Geometry: see drawing. Coordinates: mm, zero at the bounding-box minimum. A direction names the side the tool comes from. Coordinates: 2 decimals unless noted, no trailing zeros. Loops run counter-clockwise (first coordinate to the right, second up) from the corner with the lowest first, then second, coordinate; pieces in that order, holes last.
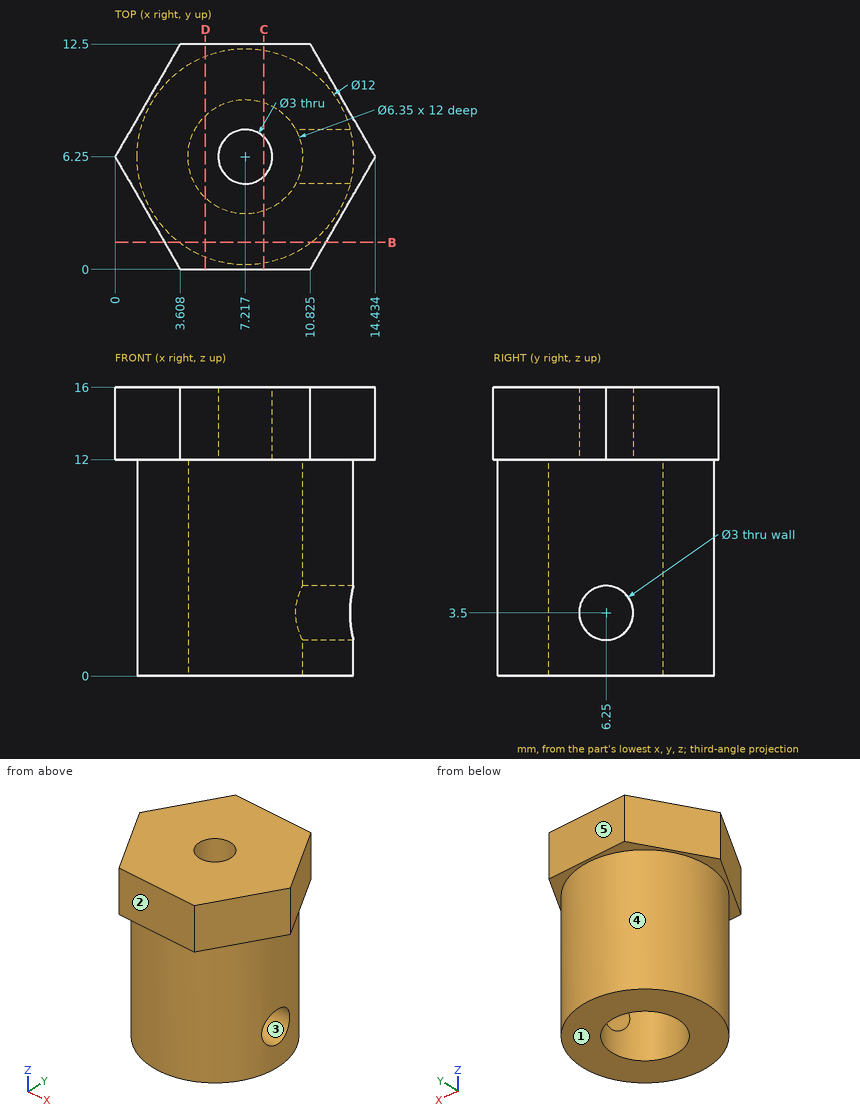
Item 1: Mould query, pull axis Z, two halves, no side actions, for the marked faces 1, 2 and 3. Classes: +Z half, -Z half, draft (parallel to the pull), parting line (faces both ways), or undercut.
Result:
face 1: -Z half
face 2: draft
face 3: undercut
Item 2: Reachability of the marked faces 4 and 5 from +Z, -Z, +X, -X, +Y, -Y: full face, straight path, thin tool, end or side. Return the list, or none.
Result:
face 4: -Z
face 5: +Z, -Z, +X, -X, +Y
Item 3: Section query B-B (y = 1.5). Output: boundary loops of the cut face in (x, z).
Result:
outline: (2.74, 12) - (3.55, 12) - (3.55, 0) - (10.88, 0) - (10.88, 12) - (11.69, 12) - (11.69, 16) - (2.74, 16) - close
Item 4: Section query D-D (x = 5). Output: boundary loops of the cut face in (y, z) (1 decimal), then the cut area to 3 significant figures.
Result:
outline: (0, 12) - (0.7, 12) - (0.7, 0) - (4, 0) - (4, 12) - (8.5, 12) - (8.5, 0) - (11.8, 0) - (11.8, 12) - (12.5, 12) - (12.5, 16) - (0, 16) - close
area: 129 mm2
Item 5: Line query: L1, parallel to X at y = 6.25, z = 6; L2, parallel to Z at x = 6.25, y = 8; L3, parallel to Y at x = 5.25, z = 6.5. Output: solid intervals per line, ascending.
Result:
L1: x = 1.22 to 4.04, 10.39 to 13.22
L2: z = 12 to 16
L3: y = 0.58 to 3.76, 8.74 to 11.92
Item 6: Contact query for flat-ended pins moving along their axis: P1, Ø1, axis at y = 10, z = 14, coming from the +X side; P2, Ø5, axis at x = 12, z = 6.5, coming from the +Y side; P3, Ø3, axis at x = 7.5, y = 5, coming from the -Z side. Output: stop coordinate, or through.
Result:
P1: stops at x = 12.56
P2: stops at y = 11.8
P3: stops at z = 12
Item 7: Section query C-C (x = 8.25). Output: boundary loops of the cut face in (y, z), then the cut area to 3 significant figures.
Result:
outline: (0, 12) - (0.34, 12) - (0.34, 0) - (3.25, 0) - (3.25, 12) - (5.16, 12) - (5.16, 16) - (0, 16) - close; (7.34, 12) - (9.25, 12) - (9.25, 0) - (12.16, 0) - (12.16, 12) - (12.5, 12) - (12.5, 16) - (7.34, 16) - close
area: 111 mm2
